```python
from build123d import *

# Parameters (mm, degrees)
F0_W      = 40
F0_H      = 20
F1_DEPTH  = 36
F2_W      = 18
F2_H      = 3
F3_DEPTH  = 7.5
F4_W      = 18
F4_H      = 2.9874
F5_DEPTH  = 7.5
F8_D      = 5
F9_R      = 7
F10_DEPTH = 1.5
F11_R     = 2.3
F12_DEPTH = 4.3
F13_R     = 1.35
F14_DEPTH = 4.9


with BuildPart() as f1:
    # F0 (on Top) → F1 (new body)
    with BuildSketch(Plane.XY):
        with Locations((0.734034, -5.869799)):
            Rectangle(F0_W, F0_H)
    extrude(amount=F1_DEPTH)

    # F2 (on face) → F3 (join)
    with BuildSketch(Plane.YZ.offset(20.734034)):
        with Locations((-5.869799, 28.848891)):
            Rectangle(F2_W, F2_H)
    extrude(amount=F3_DEPTH)

    # F4 (on face) → F5 (join)
    with BuildSketch(Plane(origin=(-19.265966, 0, 0), x_dir=(0, -1, 0), z_dir=(-1, 0, 0))):
        with Locations((5.869799, 28.855191)):
            Rectangle(F4_W, F4_H)
    extrude(amount=F5_DEPTH)

    # F8 (through all)
    with Locations(Plane.XY.offset(30.348891)):
        with Locations((-24.765966, -0.869799), (-24.838559, -11.935355), (26.234034, -10.869799), (26.234034, -0.869799)):
            Hole(F8_D / 2)

    # F9 (on face) → F10 (join)
    with BuildSketch(Plane.XY.offset(36)):
        with Locations((7.723857, -6.007267)):
            Circle(F9_R)
    extrude(amount=F10_DEPTH)

    # F11 (on face) → F12 (join)
    with BuildSketch(Plane.XY.offset(37.5)):
        with Locations((7.723857, -6.007267)):
            Circle(F11_R)
    extrude(amount=F12_DEPTH)

    # F13 (on face) → F14 (join)
    with BuildSketch(Plane.XY.offset(41.8)):
        with Locations((7.723857, -6.007267)):
            Circle(F13_R)
    extrude(amount=F14_DEPTH)


solid = f1.part
```
Source: CAD feature listing. Evaluate the final solid. Frame: model axes, mm. A direction names the side the tool comes from. Round coordinates to 2 decimals unless told otherwise and drop trailing zeros. Write each loop counter-clockwise with the first axis right and the second up, starting at its lowest first coordinate (ties: lowest second). Pieces come first, ordered by that corner, then holes. Notation, with made-up numbers: M -17.75,69.25 L 36.25,69.25 A34 cw 36.25,102.25 Z; hole C -17.5,71 d8. An arc over 180 degrees is marked long. Answer as a JSON object with one key per item and string values. Group by question number.
(1) Mould query, pull axis Y, two halves, no side actions, for faces 5 (the flat face through (-26.766, -14, 29)), 6 (the cylindrical face through (-22.267, -0.782, 28.834)), 7 (the cylindrical face through (6.21, -12.84, 36.74)). Classes: +Y half, -Y half, draft (parallel to the pull), parting line (faces both ways), or undercut.
(2) Section query D-D on x = -20.5. Output: boundary loops of the cut face in (y, z).
(3) Ray query, line 1 (Z direction, x = 3, y = -5); line 2 (X direction, y = 3.25, z = 35.5); line 3 (Z direction, x = -1.5, y = 0.75). Return the intervals inside material, ascending. Write a range as [from, to].
(4) First-contact query: pin 1 (8 mm diameter, centred on x = 26.23, y = -10.87, fed in from +Z); pin 2 (0.9 mm diameter, centred on x = 24, z = 29.5, fed in from -Y); pin 3 (8.5 mm diameter, centred on x = -24, y = -4.5, fed in from -Z). Flat tips, straight axial feed; report the tip coordinate or a pass-through.
(5) Section query A-A on x = 12. Output: boundary loops of the cut face in (y, z), then the cut area to 3 significant figures.
(6) Section query B-B on z = 34. Output: boundary loops of the cut face in (x, y).
(7) Reachability of faces 1 (the flat face through (24, 3.13, 29)), 2 (the flat face through (6, -4, 37.5)), 3 (the flat face through (24, -6, 30.349)), 4 (the flat face through (-22, -6, 30.349)) from +Z, -Z, +X, -X, +Y, -Y: full face, straight path, thin tool, end or side. Return the list, or none.
(8) Section query C-C on y = -0.25. Output: boundary loops of the cut face in (x, z).
Computed values:
{
 "1": {"face 5": "draft", "face 6": "undercut", "face 7": "parting line"},
 "2": {"outline": "M -14.87,27.36 L 3.13,27.36 L 3.13,30.35 L -14.87,30.35 Z"},
 "3": {"line 1": "[0, 37.5]", "line 2": "[-19.27, 20.73]", "line 3": "[0, 36]"},
 "4": {"pin 1": "z = 30.35", "pin 2": "y = -14.87", "pin 3": "z = 27.36"},
 "5": {"outline": "M -15.87,0 L 4.13,0 L 4.13,36 L -0.47,36 L -0.47,37.5 L -11.55,37.5 L -11.55,36 L -15.87,36 Z", "area": "737 mm^2"},
 "6": {"outline": "M -19.27,-15.87 L 20.73,-15.87 L 20.73,4.13 L -19.27,4.13 Z"},
 "7": {"face 1": "+Z, -Z, +X, +Y", "face 2": "+Z", "face 3": "+Z, +X, +Y, -Y", "face 4": "+Z, -X, +Y, -Y"},
 "8": {"outline": "M -22.34,27.36 L -19.27,27.36 L -19.27,0 L 20.73,0 L 20.73,27.35 L 23.81,27.35 L 23.81,30.35 L 20.73,30.35 L 20.73,36 L 11.71,36 L 11.71,37.5 L 3.74,37.5 L 3.74,36 L -19.27,36 L -19.27,30.35 L -22.34,30.35 Z"}
}
